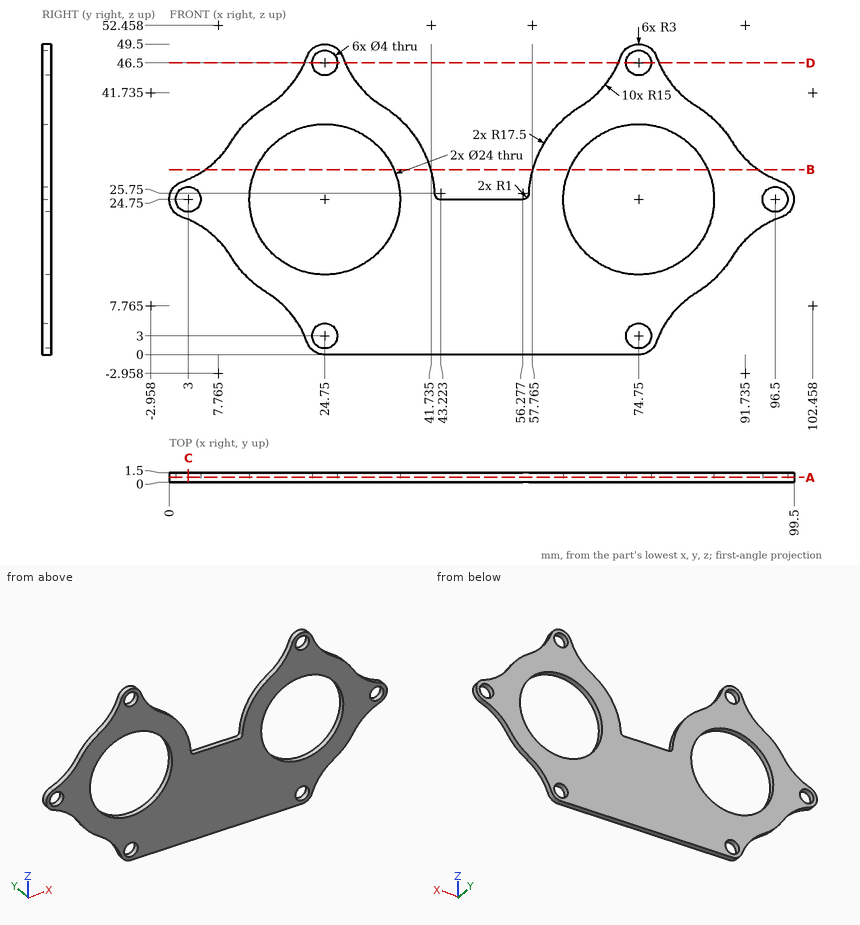
Answer from the drawing. Dimensions are ordinates in mm from the lowest x, y and z of the part. Round coordinates to 2 decimals unless told otherwise and drop trailing zeros. Loops run counter-clockwise (first coordinate to the right, second up) from the corner with the lowest first, then second, coordinate; pieces in that order, holes last. Notation, with made-up numbers: M 73,58 L 120,58 A21 cw 120,79 Z; hole C 47.25,51 d9. An arc over 180 degrees is marked long. One line per question, with ' | ' between items. Start each with the question number.
(1) Find the intervals of material crossed by line 1 (Z direction, x = 24.5, y = 1.25) (1 decimal); line 2 (X direction, y = 0.45, z = 18); line 3 (X direction, y = 0.2, z = 21), in increasing order.
(2) A flat-ended cylindrical pin translates along its axis: pin 1 Ø2.5 at (x, z) = (24.75, 46.5) entering from +Y. Find the tip coordinate at first contact, or state that the pin passes through.
(3) A cutting plane is placed at D-D on z = 46.5. Write down the section's boundary in (x, y).
(4) A cutting plane is placed at C-C on x = 3. Write down the section's boundary in (y, z).
(5) A cutting plane is placed at A-A on y = 0.75. Give the number of separate pieces and of enclosed holes in the cut face, plus the area to 3 significant figures.
(6) A cutting plane is placed at B-B on z = 29.5. Write down the section's boundary in (x, y), plus the area to 3 significant figures.
Geometry check:
1) line 1: z = 0 to 1, 5 to 12.8, 36.7 to 44.5, 48.5 to 49.5 | line 2: x = 8.01 to 14.83, 34.67 to 64.83, 84.67 to 91.49 | line 3: x = 4.1 to 13.35, 36.15 to 63.35, 86.15 to 95.4
2) pin 1: passes through
3) outline: M 21.53,0 L 22.75,0 L 22.75,1.5 L 21.53,1.5 Z; M 26.75,0 L 27.97,0 L 27.97,1.5 L 26.75,1.5 Z; M 71.53,0 L 72.75,0 L 72.75,1.5 L 71.53,1.5 Z; M 76.75,0 L 77.97,0 L 77.97,1.5 L 76.75,1.5 Z
4) outline: M 0,21.53 L 1.5,21.53 L 1.5,22.75 L 0,22.75 Z; M 0,26.75 L 1.5,26.75 L 1.5,27.97 L 0,27.97 Z
5) separate pieces: 1 | enclosed holes: 8 | area: 1,990 mm²
6) outline: M 5.72,0 L 13.73,0 L 13.73,1.5 L 5.72,1.5 Z; M 35.77,0 L 41.59,0 L 41.59,1.5 L 35.77,1.5 Z; M 57.91,0 L 63.73,0 L 63.73,1.5 L 57.91,1.5 Z; M 85.77,0 L 93.78,0 L 93.78,1.5 L 85.77,1.5 Z | area: 41.5 mm²
